Design review of the part built by this model. Coordinates are the model's own, in mm. Face numbers are marked on the shaded views. Round coordinates to 2 decimals unless told otherwise and drop trailing zeros. Order: outer loops, then holes, each group sorted by start corner. A loop starts at its lowest first (then second) coordinate and runs counter-clockwise, first axis right, second up. Notation, with made-up numbers: (0.25, -22) - (57.25, -22) arc R14 cw to (57.25, -3) - close; hole circle Ø3 at (-23.5, 65). An arc over 180 degrees is marked (long way). Write item = value, one per line.
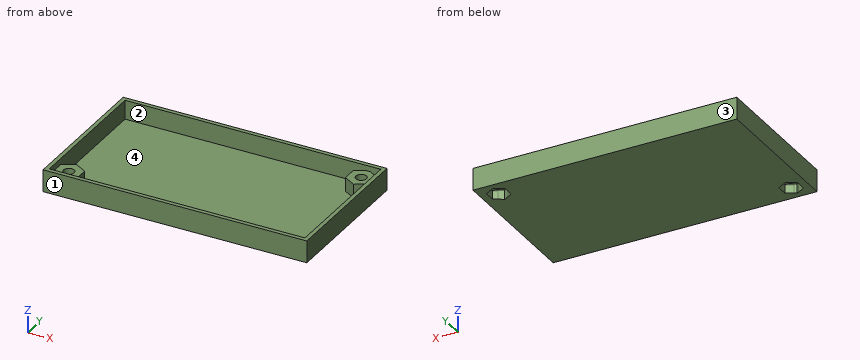
Autodesk Fusion 360 part; units mm, degrees
sketch "Sketch1" plane through (0, 0, 0) normal (0, 0, 1) x (1, 0, 0)
  line L0 (0, 0) -> (79, 0)
  line L1 (79, 0) -> (79, 44)
  line L2 (79, 44) -> (0, 44)
  line L3 (0, 44) -> (0, 0)
  line L4 (1.2, 1.2) -> (77.8, 1.2)
  line L5 (77.8, 1.2) -> (77.8, 42.8)
  line L6 (77.8, 42.8) -> (1.2, 42.8)
  line L7 (1.2, 42.8) -> (1.2, 1.2)
  line L8 (2, 42) -> (77, 42) construction
  line L9 (77, 42) -> (77, 2) construction
  line L10 (77, 2) -> (2, 2) construction
  line L11 (2, 2) -> (2, 42) construction
  circle A0 centre (74, 39) radius 1.6
  circle A1 centre (5, 5) radius 1.6
  line L12 (74, 42.2332) -> (71.2, 40.6166)
  line L13 (71.2, 40.6166) -> (71.2, 37.3834)
  line L14 (71.2, 37.3834) -> (74, 35.7668)
  line L15 (74, 35.7668) -> (76.8, 37.3834)
  line L16 (76.8, 37.3834) -> (76.8, 40.6166)
  line L17 (76.8, 40.6166) -> (74, 42.2332)
  line L18 (5, 8.2332) -> (2.2, 6.6166)
  line L19 (2.2, 6.6166) -> (2.2, 3.3834)
  line L20 (2.2, 3.3834) -> (5, 1.7668)
  line L21 (5, 1.7668) -> (7.8, 3.3834)
  line L22 (7.8, 3.3834) -> (7.8, 6.6166)
  line L23 (7.8, 6.6166) -> (5, 8.2332)
  line L24 (1.4, 2.9215) -> (5, 0.8431)
  line L25 (5, 0.8431) -> (8.6, 2.9215)
  line L26 (8.6, 2.9215) -> (8.6, 7.0785)
  line L27 (8.6, 7.0785) -> (5, 9.1569)
  line L28 (5, 9.1569) -> (1.4, 7.0785)
  line L29 (1.4, 7.0785) -> (1.4, 2.9215)
  line L30 (70.4, 36.9215) -> (74, 34.8431)
  line L31 (74, 34.8431) -> (77.6, 36.9215)
  line L32 (77.6, 36.9215) -> (77.6, 41.0785)
  line L33 (77.6, 41.0785) -> (74, 43.1569)
  line L34 (74, 43.1569) -> (70.4, 41.0785)
  line L35 (70.4, 41.0785) -> (70.4, 36.9215)
  point P0 (39.5, 42)
  point P1 (39.5, 44)
  point P2 (77, 22)
  point P3 (79, 22)
  point P4 (74, 39)
  point P5 (5, 5)
  dimension "d1" = 79
  dimension "d2" = 44
  dimension "d9" = -1.2
  dimension "d14" = 75
  dimension "d15" = 40
  dimension "d16" = 0.8
  dimension "d21" = 3.2
  dimension "d33" = 2.8
  dimension "d34" = 2.8
  dimension "d35" = 0.8
  dimension "d36" = 0.8
  dimension "d61" = 3.2
  dimension "d63" = 3
  dimension "d64" = 3
  dimension "d65" = 3
  dimension "d66" = 3
extrude "Extrude13" add sketch "Sketch1" along normal blind 5 contours L12 L13 L14 L15 L16 L17 makes body 1
extrude "Extrude14" add sketch "Sketch1" along normal blind 5 contours L6 L33 L34 | L6 L30 L31 L32 L33 L34 L35 bodies 1
extrude "Extrude15" add sketch "Sketch1" along normal blind 5 separate body contours L4 L24 L25 L26 L27 L28 L29 | L4 L24 L25 | L18 L19 L20 L21 L22 L23 makes body 2
extrude "Extrude16" add sketch "Sketch1" along normal blind 6.6 separate body contours L0 L1 L2 L3 | L4 L24 L25 | L6 L33 L34 makes body 3
extrude "Extrude17" add sketch "Sketch1" along normal blind 0.9 contours L4 L5 L6 L7 L24 L25 L26 L27 L28 L29 L30 L31 L32 L33 L34 L35 bodies 1 2 3
extrude "Extrude18" cut sketch "Sketch1" along normal blind 2.5 contours L12 L13 L14 L15 L16 L17 bodies 1
extrude "Extrude19" cut sketch "Sketch1" along normal blind 2.5 contours L18 L19 L20 L21 L22 L23 bodies 1
sketch "Sketch3" plane through (0, 0, 0) normal (0, 0, 1) x (1, 0, 0)
  line L0 (71.2, 37.4) -> (76.8, 37.4)
  line L1 (76.8, 37.4) -> (74, 35.7468)
  line L2 (74, 35.7468) -> (71.2, 37.4)
  line L3 (71.2, 40.6) -> (76.8, 40.618)
  line L4 (71.2, 40.6) -> (74, 42.2444)
  line L5 (74, 42.2444) -> (76.8, 40.618)
  line L6 (71.2, 37.4) -> (72.4601, 37.4)
  line L7 (2.2, 3.4) -> (7.8, 3.4)
  line L8 (7.8, 3.4) -> (5, 1.7617)
  line L9 (5, 1.7617) -> (2.2, 3.4)
  line L10 (2.2, 6.6) -> (4.9648, 8.2176)
  line L11 (4.9648, 8.2176) -> (7.8, 6.6)
  line L12 (7.8, 6.6) -> (2.2, 6.6)
extrude "Extrude20" cut sketch "Sketch3" along normal blind 2.8 contours L7 L8 L9 | L10 L11 L12 bodies 1
extrude "Extrude21" cut sketch "Sketch3" along normal blind 2.8 contours L0 L1 L2 L6 | L3 L4 L5 bodies 1
equation "d1 = TotalDepth"
equation "d2 = TotalWidth"
equation "LayerHeight = 0.3 mm"
equation "Tolerance = 0.1 mm"
equation "ExtrusionWidth = 0.4 mm"
equation "TotalWidth = 44 mm"
equation "TotalDepth = 79 mm"
equation "TotalHeight = 35 mm"
equation "d9 = -3 * ExtrusionWidth"
equation "PCBWidth = 75 mm"
equation "PCBLength = 40 mm"
equation "PCBThickness = 1.6 mm"
equation "PCBSolderingHeight = 4 mm"
equation "d14 = PCBWidth"
equation "d15 = PCBLength"
equation "d21 = M3Adjusted"
equation "M3Adjusted = 3 mm + Tolerance * 2"
equation "PCBSupportHeight = PCBSolderingHeight + Tolerance + BaseThickness"
equation "BottomCaseHeight = PCBSolderingHeight + Tolerance + PCBThickness + BaseThickness"
equation "NutWidth = 5.5 mm + Tolerance"
equation "NutHeight = 2.4 mm + Tolerance"
equation "d33 = NutWidth / 2"
equation "d34 = NutWidth / 2"
equation "d35 = 2 * ExtrusionWidth"
equation "d36 = 2 * ExtrusionWidth"
equation "NutSupportHeight = NutHeight + Tolerance + BaseThickness"
equation "BaseThickness = 3 * LayerHeight"
equation "HoleSpreading = PCBHoleSpread + M3Adjusted / 2"
equation "d61 = M3Adjusted"
equation "PCBHoleSpread = 1.40 mm"
equation "d63 = HoleSpreading"
equation "d64 = HoleSpreading"
equation "d65 = HoleSpreading"
equation "d66 = HoleSpreading"
equation "d67 = PCBSupportHeight"
equation "d69 = PCBSupportHeight"
equation "d71 = PCBSupportHeight"
equation "d73 = BottomCaseHeight"
equation "d75 = BaseThickness"
equation "d77 = NutHeight"
equation "d79 = NutHeight"
equation "d82 = NutHeight + LayerHeight"
equation "d84 = NutHeight + LayerHeight"
properties part number "Configuration1"
1) We need section A-A on y = 39. Write out the cut boundary in (x, z), and give its area (3 significant figures).
Findings:
outline = (0, 0) - (71.2, 0) - (71.2, 2.5) - (72.4, 2.5) - (72.4, 5) - (70.4, 5) - (70.4, 0.9) - (1.2, 0.9) - (1.2, 6.6) - (0, 6.6) - close; (75.6, 2.5) - (76.8, 2.5) - (76.8, 0) - (79, 0) - (79, 6.6) - (77.8, 6.6) - (77.8, 0.9) - (77.6, 0.9) - (77.6, 5) - (75.6, 5) - close
area = 92.3 mm^2
2) We need section C-C on y = 11. Write out the cut boundary in (x, z), and give its area (3 significant figures).
Findings:
outline = (0, 0) - (79, 0) - (79, 6.6) - (77.8, 6.6) - (77.8, 0.9) - (1.2, 0.9) - (1.2, 6.6) - (0, 6.6) - close
area = 84.8 mm^2
3) The part is to be moulded in two halves that separate along Y. For the marked faces 1, 2, 3 and 4, say which applies: released by +Y, released by -Y, zero draft, split by the parting line, or undercut.
Findings:
face_1 = released by -Y
face_2 = undercut
face_3 = released by +Y
face_4 = undercut
4) To check wall thickness, follow L1, parallel to X at y = 39, z = 4.25; L2, parallel to Y at x = 74, z = 3.55; L3, parallel to X at y = 7, z = 3.5. State the ranges of each line that lie inside material, in increasing order. Write a range as from..to.
Findings:
L1 = 0..1.2, 70.4..72.4, 75.6..77.6, 77.8..79
L2 = 0..1.2, 34.84..37.4, 40.6..44
L3 = 0..1.2, 1.4..8.6, 77.8..79
5) We need section B-B on x = 63. Write out the cut boundary in (y, z), and give its area (3 significant figures).
Findings:
outline = (0, 0) - (44, 0) - (44, 6.6) - (42.8, 6.6) - (42.8, 0.9) - (1.2, 0.9) - (1.2, 6.6) - (0, 6.6) - close
area = 53.3 mm^2
6) Clearance check with flat-ended pins moving along their axes: pin 1 Ø0.8 at (x, y) = (3.5, 4.5) entering from -Z; pin 2 Ø1 at (y, z) = (13.5, 5) entering from -X; pin 3 Ø6 at (x, y) = (62.5, 23.5) entering from +Z; pin 4 Ø3.5 at (x, y) = (5, 5) entering from +Z. State where each tip first meets the part, or that it passes through.
Findings:
pin_1 = 2.5
pin_2 = 0
pin_3 = 0.9
pin_4 = 5
